The model under review builds one solid part; all positions refer to its coordinate system, in mm. Face numbers are marked on the shaded views. A direction names the side the tool comes from. Give positions to 0.01 mm unless a question says otherwise; leave off trailing zeros. Order: outer loops, then holes, each group sorted by start corner. A loop starts at its lowest first (then second) coordinate and runs counter-clockwise, first axis right, second up. Notation, with made-up numbers: M -14.5,-15 L 15.5,-15 A17 ccw 15.5,-10 Z; hole C 68.5,-15 d7. An arc over 180 degrees is marked long. One line per question, with ' | ' between items. Start each with the question number.
1. For the marked faces 4 and 5, list the 3-axis set-ups (+Z, -Z, +X, -X, +Y, -Y) from which the entire face can be reached by the end or side of a thin tool; tool diameter is ignored.
2. We need section A-A on z = -33. Write out the cut boundary in (x, y).
3. Insertion check: P1, Ø1, axis at y = -10.5, z = 35.5, coming from the +X side; P2, Ø5, axis at x = -4, z = 3.5, coming from the +Y side; P3, Ø10, axis at x = -12, y = 8, coming from the +Z side (3 decimals); P4, Ø3, axis at x = -1.5, z = 4.5, coming from the -Y side. Each pin has a flat end and moves straight along its axis. Give the tip position at first contact, or say it passes through.
4. Wall thickness on L1, parallel to Z at x = -23, y = -1.5; L2, parallel to Z at x = 0, y = -17; L3, parallel to Y at x = -15.5, z = 52: over which ranges is each line inside the solid? List them lowest first.
5. We need section B-B on z = 30. Write out the cut boundary in (x, y).
6. The part is to be moulded in two halves that separate along Z. For the marked faces 1, 2 and 3, say which applies: +Z half, -Z half, draft (parallel to the pull), parting line (faces both ways), or undercut.
```python
from build123d import *

# Parameters (mm, degrees)
F2_W          = 30.5360297733
F2_H          = 20.1705897587
F3_DEPTH      = 25.401
F3_DEPTH_BACK = 25.4
F4_R          = 1.5875
F5_SIZE       = 1.6002
F6_R          = 19.05
F7_R          = 5.08


with BuildPart() as f1:
    # F0 (on Front) → F1 (revolve)
    with BuildSketch(Plane.XZ):
        with BuildLine():
            Line((-25.4, 0), (-12.7, 0))
            Line((-12.7, 0), (-12.7, -55.5625))
            Line((-12.7, -55.5625), (0, -55.5625))
            Line((0, -55.5625), (0, 0))
            Line((0, 0), (0, 7.9375))
            Line((0, 7.9375), (0, 19.05))
            Line((0, 19.05), (0, 66.675))
            Line((0, 66.675), (-12.2967221242, 66.675))
            ThreePointArc((-12.2967221242, 66.675), (-25.3989438933, 44.6816227592), (-12.7, 22.4529547439))
            Line((-12.7, 22.4529547439), (-12.7, 7.9375))
            Line((-12.7, 7.9375), (-25.4, 7.9375))
            Line((-25.4, 7.9375), (-25.4, 0))
        make_face()
    revolve(axis=Axis((0, 0, -27.78125), (0, 0, -1)))

    # F2 (on Right) → F3 (cut, two sides)
    with BuildSketch(Plane.YZ) as f3_sk:
        with Locations((-34.3180148866, 4.7039177944)):
            Rectangle(F2_W, F2_H)
        with Locations((34.3180148866, 4.7039177944)):
            Rectangle(F2_W, F2_H)
    extrude(amount=-F3_DEPTH, mode=Mode.SUBTRACT)
    extrude(f3_sk.sketch, amount=F3_DEPTH_BACK, mode=Mode.SUBTRACT)

    # F4
    f4_edges = [f1.edges().sort_by_distance(p)[0] for p in [
        (-25.4, 0, 7.9375),
        (25.4, 0, 7.9375),
        (0, -19.05, 7.9375),
        (0, 19.05, 7.9375),
        (16.800521, 19.05, 3.96875),
        (-16.800521, 19.05, 3.96875),
        (16.800521, -19.05, 3.96875),
        (-16.800521, -19.05, 3.96875),
    ]]
    fillet(f4_edges, radius=F4_R)

    # F5
    f5_edges = [f1.edges().sort_by_distance(p)[0] for p in [
        (12.7, 0, -55.5625),
    ]]
    chamfer(f5_edges, length=F5_SIZE)

    # F6
    f6_edges = [f1.edges().sort_by_distance(p)[0] for p in [
        (12.7, 0, 22.452955),
    ]]
    fillet(f6_edges, radius=F6_R)

    # F7
    f7_edges = [f1.edges().sort_by_distance(p)[0] for p in [
        (12.7, 0, 7.9375),
    ]]
    fillet(f7_edges, radius=F7_R)


solid = f1.part
```
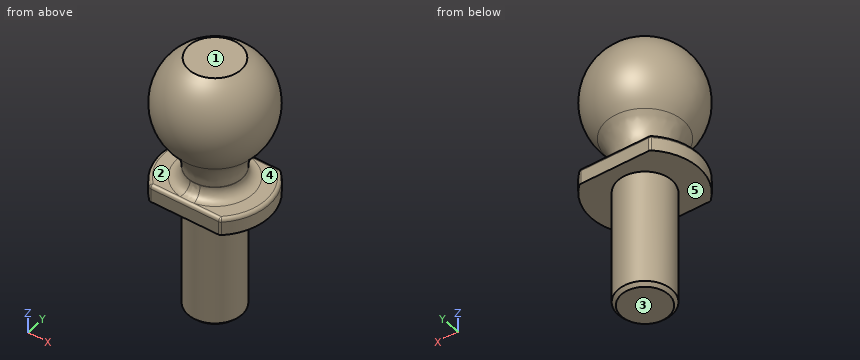
Entries:
1) face 4: +X | face 5: -Z
2) outline: C 0,0 d25.4
3) P1: stops at x = 21.64 | P2: stops at y = 19.05 | P3: stops at z = 66.675 | P4: stops at y = -19.05
4) L1: z = 0 to 7.94, 33.78 to 55.12 | L2: z = 0 to 7.99, 25.4 to 63.32 | L3: y = -18.65 to 18.65
5) outline: C 0,0 d41.78
6) face 1: +Z half | face 2: undercut | face 3: -Z half
